Source: CAD feature listing. Evaluate the final solid. Frame: model axes, mm. Face numbers are marked on the shaded views. A direction names the side the tool comes from. Give positions to 0.01 mm unless a question says otherwise; leave off trailing zeros. Order: outer loops, then holes, each group sorted by start corner. A loop starts at its lowest first (then second) coordinate and runs counter-clockwise, first axis right, second up.
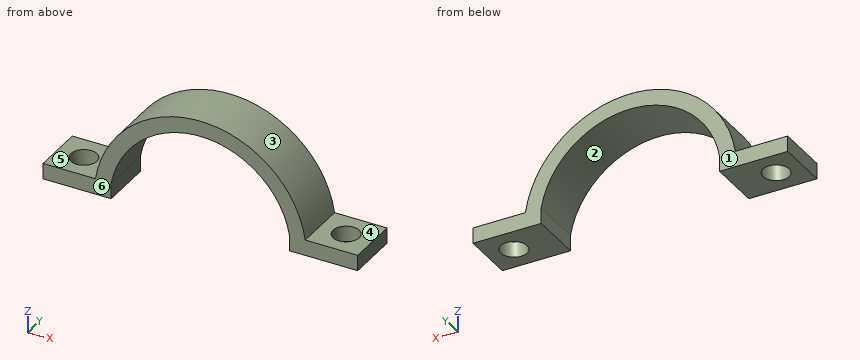
from build123d import *

# Parameters (mm, degrees)
PAD_DEPTH    = 10
SKETCH001_R  = 2.5
POCKET_DEPTH = 3


with BuildPart() as part:
    # Sketch → Pad (new body)
    with BuildSketch(Plane.XZ):
        with BuildLine():
            Line((-30, 0), (-17, 0))
            Line((-17, 3), (-17, 0))
            ThreePointArc((17, 3), (0, 17.262677), (-17, 3))
            Line((17, 3), (17, 0))
            Line((17, 0), (30, 0))
            Line((30, 0), (30, 3))
            Line((30, 3), (20, 3))
            ThreePointArc((20, 3), (0, 20.223748), (-20, 3))
            Line((-30, 3), (-20, 3))
            Line((-30, 0), (-30, 3))
        make_face()
    extrude(amount=PAD_DEPTH)

    # Sketch001 (on Face8 of Pad) → Pocket (cut)
    with BuildSketch(Plane(origin=(0, 0, 3), x_dir=(-1, 0, 0), z_dir=(0, 0, 1))):
        with Locations((25, 5)):
            Circle(SKETCH001_R)
        with Locations((-25, 5)):
            Circle(SKETCH001_R)
    extrude(amount=-POCKET_DEPTH, mode=Mode.SUBTRACT)


solid = part.part
(1) Access query for the marked faces 4, 5 and 6. Directions: +Z, -Z, +X, -X, +Y, -Y. A direction counts if a zero-diameter tool reaches every point of the face in a straight line with its end or side. Return the directions, or none.
(2) Section A-A, the plane x = -23.5. Return loops of the section in (y, z), plus the area to 3 significant figures.
(3) Section B-B, the plane y = -3.5. Return loops of the section in (x, z), plus the area to 3 significant figures.
(4) Section D-D, the plane y = -8.25. Return loops of the section in (x, z).
(5) Pin query (flat end, axial travel): pin 1 Ø1 at (x, y) = (-22.5, -1) entering from -Z; pin 2 Ø6 at (x, y) = (-21, -3) entering from +Z; pin 3 Ø6 at (x, y) = (5.5, -7.5) entering from -Z (3 decimals). Return the tip coordinate at first contact, or that it passes through.
(6) Draft query along X for the marked faces 1, 2 and 3. Return one class per face: +X half, -X half, draft (parallel to the pull), parting line (faces both ways), or undercut.
(7) Line query: line 1 along X through (y, z) = (-5, 2.35); line 2 along Y through (x, z) = (-25, 0.8); line 3 along X through (y, z) = (-5.75, 3.75). Output: solid intervals per line, ascending.
(8) Section C-C, the plane z = 6.5. Return loops of the section in (x, y).
Checks:
1. face 4: +Z, +X, +Y, -Y
1. face 5: +Z, -X, +Y, -Y
1. face 6: +Z, -Z, +X, -X, -Y
2. outline: (-10, 0) - (-7, 0) - (-7, 3) - (-10, 3) - close; (-3, 0) - (0, 0) - (0, 3) - (-3, 3) - close
2. area: 18.0 mm2
3. outline: (-30, 0) - (-27, 0) - (-27, 3) - (-30, 3) - close; (-23, 0) - (-17, 0) - (-17, 3) arc R17.26 cw to (17, 3) - (17, 0) - (23, 0) - (23, 3) - (20, 3) arc R20.22 ccw to (-20, 3) - (-23, 3) - close; (27, 0) - (30, 0) - (30, 3) - (27, 3) - close
3. area: 211 mm2
4. outline: (-30, 0) - (-17, 0) - (-17, 3) arc R17.26 cw to (17, 3) - (17, 0) - (30, 0) - (30, 3) - (20, 3) arc R20.22 ccw to (-20, 3) - (-30, 3) - close
5. pin 1: stops at z = 0
5. pin 2: stops at z = 9.22
5. pin 3: stops at z = 15.025
6. face 1: draft
6. face 2: undercut
6. face 3: parting line
7. line 1: x = -30 to -27.5, -22.5 to -17, 17 to 22.5, 27.5 to 30
7. line 2: y = -10 to -7.5, -2.5 to 0
7. line 3: x = -19.87 to -16.85, 16.85 to 19.87
8. outline: (-19.15, -10) - (-15.99, -10) - (-15.99, 0) - (-19.15, 0) - close; (15.99, -10) - (19.15, -10) - (19.15, 0) - (15.99, 0) - close
